Could you check a few things on this drawing? It's one solid part, dimensions in mm from its lowest x, y, z. A direction names the side the tool comes from. Give positions to 0.01 mm unless a question says otherwise; leave off trailing zeros. Loops run counter-clockwise (first coordinate to the right, second up) from the corner with the lowest first, then second, coordinate; pieces in that order, holes last. Notation, with made-up numbers: M 31,38 L 53,38 A20 cw 53,46 Z; hole C 88.5,14 d2. An arc over 180 degrees is marked long. Answer in a Markdown table with one row per item. Add a question column.
1. If we section it at A-A on x = 1.27: List the corners of the cut face in (y, z) for me.
2. If we section it at B-B on z = 2: List the corners of the cut face in (x, y) for me.
3. I need wall thicknesses on line 1 along Z through (x, y) = (13.25, 2.1); line 2 along X through (y, z) = (0.35, 3.25); line 3 along X through (y, z) = (0.3, 4.25). Which ranges of each line are inside material? Lowest first, please. Write a range as from..to.
4. Thinking about a two-plate mould opening in X: for the marked faces 1, 2 and 3, which applies, released by +X, released by -X, zero draft, split by the parting line, or undercut?
5. I'm going to push a flat-ended pin straight in: pin 1 Ø1.5 at (x, y) = (6.5, 0.5) entering from -Z. Where does the tip first touch, or does it pass through?
6. If we section it at C-C on z = 0.75: List the corners of the cut face in (x, y) for me.
7. If we section it at D-D on y = 0.65: List the corners of the cut face in (x, z) for me (1 decimal).
8. Which directions (+Z, -Z, +X, -X, +Y, -Y) give clear straight access to the entire face, cutting with the end or side of a thin tool? Please do the marked faces 4 and 5.
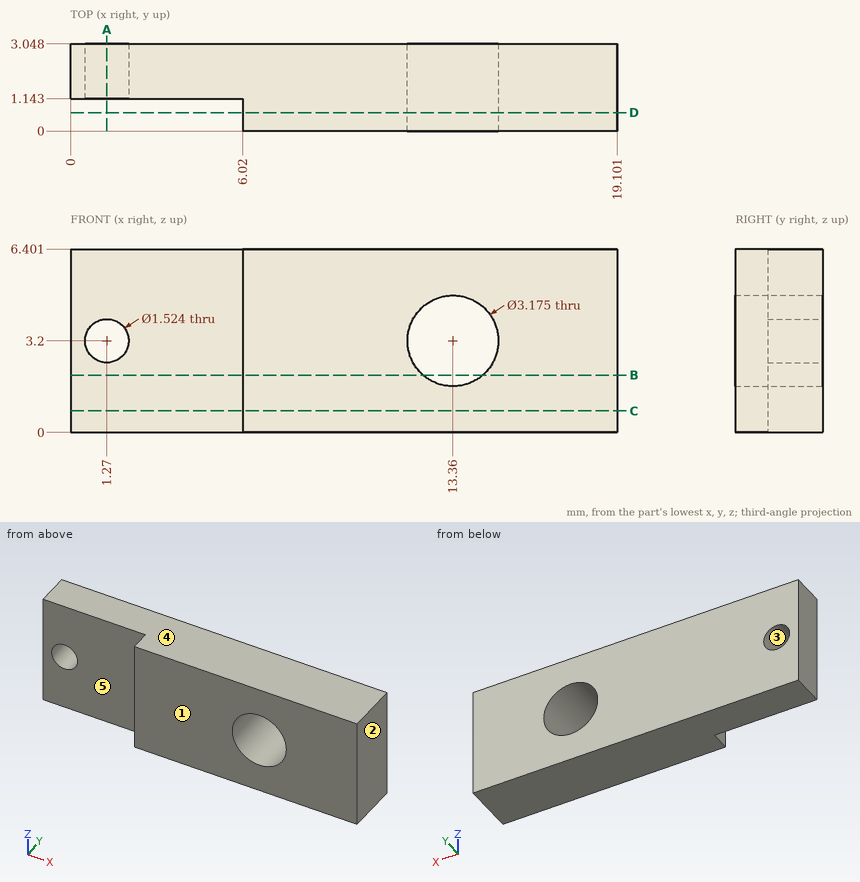
Results:
| question | item | result |
|---|---|---|
| 1 | outline | M 1.14,0 L 3.05,0 L 3.05,2.44 L 1.14,2.44 Z; M 1.14,3.96 L 3.05,3.96 L 3.05,6.4 L 1.14,6.4 Z |
| 2 | outline | M 0,1.14 L 6.02,1.14 L 6.02,0 L 12.32,0 L 12.32,3.05 L 0,3.05 Z; M 14.4,0 L 19.1,0 L 19.1,3.05 L 14.4,3.05 Z |
| 3 | line 1 | 0..1.62, 4.78..6.4 |
| 3 | line 2 | 6.02..11.77, 14.95..19.1 |
| 3 | line 3 | 6.02..12.17, 14.55..19.1 |
| 4 | face 1 | zero draft |
| 4 | face 2 | released by +X |
| 4 | face 3 | undercut |
| 5 | pin 1 | z = 0 |
| 6 | outline | M 0,1.14 L 6.02,1.14 L 6.02,0 L 19.1,0 L 19.1,3.05 L 0,3.05 Z |
| 7 | outline | M 6,0 L 19.1,0 L 19.1,6.4 L 6,6.4 Z; hole C 13.4,3.2 d3.2 |
| 8 | face 4 | +Z, +X, -X, +Y, -Y |
| 8 | face 5 | +Z, -Z, -X, -Y |
